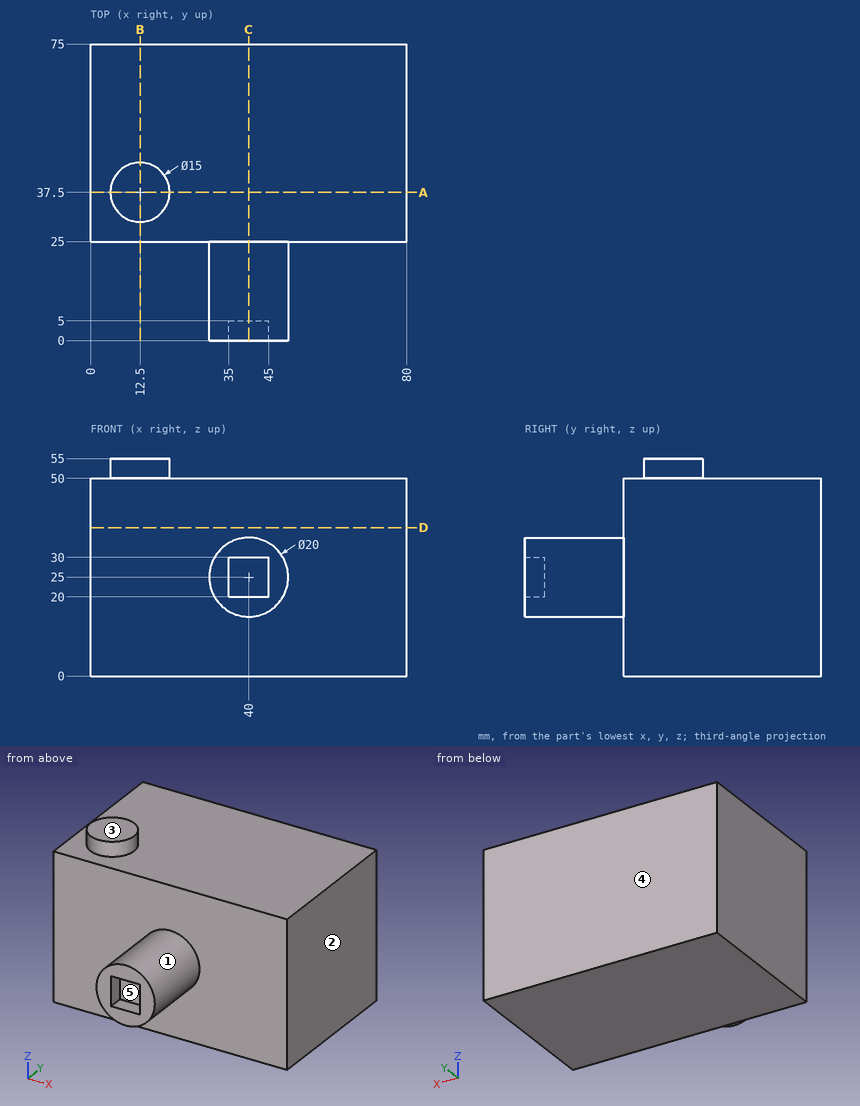
Input: dimensioned drawing with shaded views. Units: mm. Origin: part minimum x, y, z. A direction names the side the tool comes from. Round coordinates to 2 decimals unless told otherwise and drop trailing zeros. Loops run counter-clockwise (first coordinate to the right, second up) from the corner with the lowest first, then second, coordinate; pieces in that order, holes last. Notation, with made-up numbers: M 8.25,69.25 L 40.25,69.25 A21 cw 40.25,85.25 Z; hole C 75.25,-8 d6. An arc over 180 degrees is marked long. Answer in a Markdown table with one row per item. Add a question column.
1. Contact query for flat-ended pins moving along their axis: pin 1 (5 mm diameter, centred on x = 39.5, z = 25, fed in from -Y); pin 2 (1.5 mm diameter, centred on x = 43, z = 8.5, fed in from -Y); pin 3 (1.5 mm diameter, centred on x = 14, y = 45.5, fed in from -Z); pin 4 (1.5 mm diameter, centred on y = 1.5, z = 25.5, fed in from -X). Output: stop coordinate, or through.
2. Section A-A (y = 37.5). Output: boundary loops of the cut face in (x, z).
3. Set-up query: the marked faces 1 and 2. Return all of +Z, -Z, +X, -X, +Y, -Y with unobstructed straight access to the full face (end or side cutting, diameter ignored); none if empty.
4. Section D-D (z = 37.5). Output: boundary loops of the cut face in (x, y).
5. Section B-B (x = 12.5). Output: boundary loops of the cut face in (y, z).
6. Ray query, probe 1 along Z at (x, y) = (34, 58); probe 2 along Y at (x, z) = (26, 46); probe 3 along Y at (x, z) = (36.5, 24.5). Return the intervals inside material, ascending.
7. Section C-C (x = 40). Output: boundary loops of the cut face in (y, z), and give its area (3 significant figures).
8. Mould query, pull axis Z, two halves, no side actions, for the marked faces 3, 4 and 5. Classes: released by +Z, released by -Z, zero draft, split by the parting line, or undercut.
Values follow:
| question | item | result |
|---|---|---|
| 1 | pin 1 | y = 5 |
| 1 | pin 2 | y = 25 |
| 1 | pin 3 | z = 0 |
| 1 | pin 4 | x = 30 |
| 2 | outline | M 0,0 L 80,0 L 80,50 L 20,50 L 20,55 L 5,55 L 5,50 L 0,50 Z |
| 3 | face 1 | -Y |
| 3 | face 2 | +Z, -Z, +X, +Y, -Y |
| 4 | outline | M 0,25 L 80,25 L 80,75 L 0,75 Z |
| 5 | outline | M 25,0 L 75,0 L 75,50 L 45,50 L 45,55 L 30,55 L 30,50 L 25,50 Z |
| 6 | probe 1 | 0 to 50 |
| 6 | probe 2 | 25 to 75 |
| 6 | probe 3 | 5 to 75 |
| 7 | outline | M 0,15 L 25,15 L 25,0 L 75,0 L 75,50 L 25,50 L 25,35 L 0,35 L 0,30 L 5,30 L 5,20 L 0,20 Z |
| 7 | area | 2,950 mm^2 |
| 8 | face 3 | released by +Z |
| 8 | face 4 | zero draft |
| 8 | face 5 | undercut |
